Geometry: final body of the model. Coordinates: model frame, mm. Face numbers are marked on the shaded views. A direction names the side the tool comes from. Give positions to 0.01 mm unless a question says otherwise; leave off trailing zeros. Loops run counter-clockwise (first coordinate to the right, second up) from the corner with the lowest first, then second, coordinate; pieces in that order, holes last. Notation, with made-up numbers: (58.5, -40) - (107.5, -40) arc R20 ccw to (107.5, -25) - close; hole circle Ø3 at (-37.75, 18.25). An arc over 180 degrees is marked (long way). Use CSV: the item, a comma, the result in double quotes. Start each with the question number.
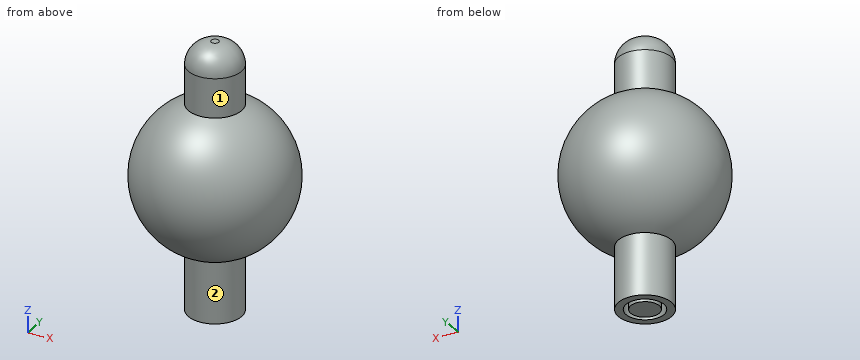
```python
from build123d import *

# Parameters (mm, degrees)
F0_R     = 7
F0_R_2   = 5
F0_R_3   = 3.75
F1_DEPTH = 70
F4_DEPTH = 35
F5_R     = 6


with BuildPart() as f1:
    # F0 (on Top) → F1 (new body)
    with BuildSketch(Plane.XY):
        Circle(F0_R)
        Circle(F0_R_2, mode=Mode.SUBTRACT)
        Circle(F0_R_2)
        Circle(F0_R_3, mode=Mode.SUBTRACT)
        Circle(F0_R_3)
    extrude(amount=F1_DEPTH)

    # F2 (on Front) → F3 (revolve)
    with BuildSketch(Plane.XZ):
        with BuildLine():
            ThreePointArc((0, 55), (-20, 35), (0, 15))
            Line((0, 15), (0, 55))
        make_face()
    revolve(axis=Axis((0, 0, 35), (0, 0, 1)))

    # F0 (on Top) → F4 (cut)
    with BuildSketch(Plane.XY):
        Circle(F0_R_2)
        Circle(F0_R_3, mode=Mode.SUBTRACT)
    extrude(amount=F4_DEPTH, mode=Mode.SUBTRACT)

    # F5
    f5_edges = [f1.edges().sort_by_distance(p)[0] for p in [
        (-7, 0, 70),
    ]]
    fillet(f5_edges, radius=F5_R)


solid = f1.part
```
Item 1: Section C-C (y = -9). Output: boundary loops of the cut face in (x, z).
Item 2: Section B-B (x = -14). Output: boundary loops of the cut face in (y, z), plus the area to 3 significant figures.
Item 3: Reachability of the marked faces 1 and 2 from +Z, -Z, +X, -X, +Y, -Y: full face, straight path, thin tool, end or side. Return the list, or none.
Item 4: Section D-D (z = 25). Output: boundary loops of the cut face in (x, y).
Item 5: Pin query (flat end, axial travel): pin 1 Ø2 at (x, z) = (2, 59.5) entering from +Y; pin 2 Ø8 at (x, z) = (-6, 35) entering from +Y; pin 3 Ø1 at (x, y) = (6, 9.5) entering from +Z. Return the tip coordinate at first contact, or that it passes through.
Item 6: Ray query, probe 1 along Y at (x, z) = (0, 13); probe 2 along Y at (x, z) = (0, 28) (3 decimals); probe 3 along X at (y, z) = (-1, 18.5). Return the intervals inside material, ascending.
Item 7: Section A-A (z = 11). Output: boundary loops of the cut face in (x, y).
Outcome:
1,outline,"circle Ø35.72 at (0, 35)"
2,outline,"circle Ø28.57 at (0, 35)"
2,area,"641 mm2"
3,face 1,"+Z"
3,face 2,"-Z"
4,outline,"circle Ø34.64 at (0, 0); circle Ø7.5 at (0, 0); hole circle Ø10 at (0, 0)"
5,pin 1,"stops at y = 6.93"
5,pin 2,"stops at y = 19.9"
5,pin 3,"stops at z = 51.87"
6,probe 1,"y = -7 to -5, -3.75 to 3.75, 5 to 7"
6,probe 2,"y = -18.735 to -5, -3.75 to 3.75, 5 to 18.735"
6,probe 3,"x = -11.26 to -4.9, -3.61 to 3.61, 4.9 to 11.26"
7,outline,"circle Ø14 at (0, 0); circle Ø7.5 at (0, 0); hole circle Ø10 at (0, 0)"
